The listing builds one solid part. Answer for the finished solid, in the listing's coordinates (mm). Face numbers are marked on the shaded views. A direction names the side the tool comes from. Give positions to 0.01 mm unless a question says otherwise; leave off trailing zeros. Order: outer loops, then holes, each group sorted by start corner. A loop starts at its lowest first (then second) coordinate and runs counter-clockwise, first axis right, second up. Notation, with made-up numbers: M 77.25,-24.5 L 121.25,-24.5 A3 cw 121.25,-20.5 Z; hole C 83,11.5 d10. An arc over 180 degrees is marked long. Answer as a JSON object with one key per item and string values. Group by question number.
```python
from build123d import *

# Parameters (mm, degrees)
SKETCH1_R           = 3.99
BOSS_EXTRUDE1_DEPTH = 16
BOSS_EXTRUDE7_DEPTH = 15
SKETCH7_R           = 3.99
BOSS_EXTRUDE8_DEPTH = 15


with BuildPart() as part:
    # Sketch1 → Boss-Extrude1 (new body)
    with BuildSketch(Plane.XY):
        with Locations((-14.383915809, -0.854852817)):
            Circle(SKETCH1_R)
    extrude(amount=BOSS_EXTRUDE1_DEPTH)

    # Sketch6 → Boss-Extrude7 (add)
    with BuildSketch(Plane.XY.offset(16)):
        with BuildLine():
            Line((-17.383915809, 2.084534875), (-17.383915809, 8.084534875))
            Line((-17.383915809, 8.084534875), (-11.383915809, 8.084534875))
            Line((-11.383915809, 8.084534875), (-11.383915809, 2.084534875))
            ThreePointArc((-11.383915809, 2.084534875), (-14.383915809, -5.054852817), (-17.383915809, 2.084534875))
        make_face()
    extrude(amount=BOSS_EXTRUDE7_DEPTH)

    # Sketch7 → Boss-Extrude8 (add)
    with BuildSketch(Plane.XY.offset(31)):
        with Locations((-14.383915809, -0.854852817)):
            Circle(SKETCH7_R)
    extrude(amount=BOSS_EXTRUDE8_DEPTH)


solid = part.part
```
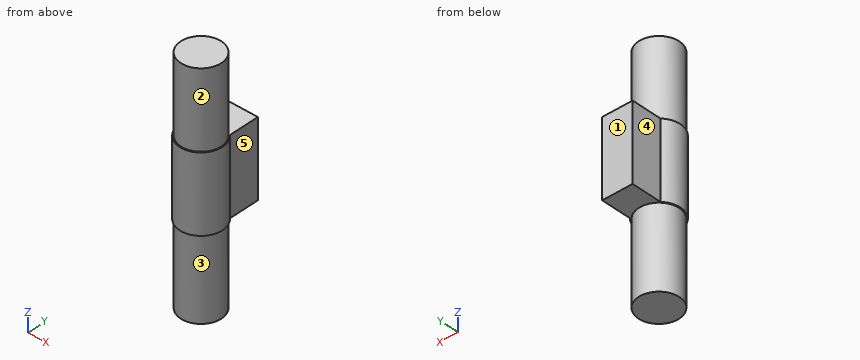
Item 1: Section C-C (z = 18.5) is taken. Determine the outline of the cut face in (x, y), and give its area (3 significant figures).
Item 2: Section B-B (y = -4) is taken. Determine the outline of the cut face in (x, z), and give its area (3 significant figures).
Item 3: A tool of negligible diameter and unlimited length cuts with its end or side. For the marked faces 1, 2, 3, 4 and 5, from which of +Z, -Z, +X, -X, +Y, -Y can it reach the whole face along a straight path? Write none if from no direction.
Item 4: Section D-D (y = 5.75) is taken. Determine the outline of the cut face in (x, z).
Item 5: Flat-ended cylindrical pins translate along their axes: P1, Ø1.5, axis at x = -16.5, z = 18.5, coming from the -Y side; P2, Ø1.8, axis at y = 4, z = 25.5, coming from the +X side; P3, Ø2, axis at y = -1.5, z = 21, coming from the +X side; P4, Ø5, axis at y = 2, z = 40, coming from the +X side. Find the tip coordinate at first contact, or state that the pin passes through.
Item 6: Consider probe 1 along X at (y, z) = (4.75, 26); probe 2 along Z at (x, y) = (-16.5, 5.25); probe 3 along X at (y, z) = (-0.75, 18.5). Determine where each line is inside the solid, lowest interval first. Write a range as from..to.
Item 7: Section A-A (x = -16) is taken. Determine the outline of the cut face in (y, z).
Values found:
{
 "1": {"outline": "M -17.38,2.08 A4.2 ccw long -11.38,2.08 L -11.38,8.08 L -17.38,8.08 Z", "area": "86.2 mm^2"},
 "2": {"outline": "M -17.17,16 L -16.84,16 L -16.84,0 L -11.93,0 L -11.93,16 L -11.6,16 L -11.6,31 L -11.93,31 L -11.93,46 L -16.84,46 L -16.84,31 L -17.17,31 Z", "area": "236 mm^2"},
 "3": {"face 1": "+Z, -Z, +X, -X, +Y", "face 2": "+Z", "face 3": "-Z", "face 4": "+Z, -Z, -X, +Y", "face 5": "+Z, -Z, +X, +Y"},
 "4": {"outline": "M -17.38,16 L -11.38,16 L -11.38,31 L -17.38,31 Z"},
 "5": {"P1": "stops at y = -4.83", "P2": "stops at x = -11.38", "P3": "stops at x = -10.18", "P4": "stops at x = -10.41"},
 "6": {"probe 1": "x = -17.38..-11.38", "probe 2": "z = 16..31", "probe 3": "x = -18.58..-10.19"},
 "7": {"outline": "M -4.73,16 L -4.5,16 L -4.5,0 L 2.79,0 L 2.79,16 L 8.08,16 L 8.08,31 L 2.79,31 L 2.79,46 L -4.5,46 L -4.5,31 L -4.73,31 Z"}
}
